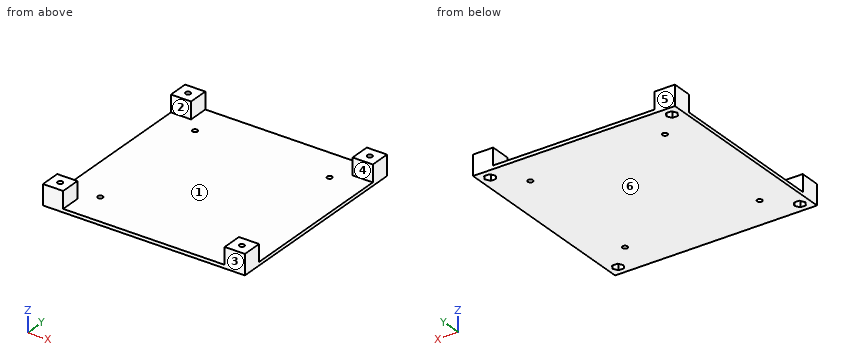
from build123d import *

# Parameters (mm, degrees)
SKETCH_W     = 120
SKETCH_H     = 120
SKETCH_R     = 1.5
PAD_DEPTH    = 2
SKETCH002_W  = 12
SKETCH002_H  = 12
SKETCH002_R  = 1.5
PAD001_DEPTH = 12
POCKET_DEPTH = 9


with BuildPart() as part:
    # Sketch → Pad (new body)
    with BuildSketch(Plane.XY):
        Rectangle(SKETCH_W, SKETCH_H)
        with Locations((-40, 40)):
            Circle(SKETCH_R, mode=Mode.SUBTRACT)
        with Locations((40, 40)):
            Circle(SKETCH_R, mode=Mode.SUBTRACT)
        with Locations((40, -40)):
            Circle(SKETCH_R, mode=Mode.SUBTRACT)
        with Locations((-40, -40)):
            Circle(SKETCH_R, mode=Mode.SUBTRACT)
        with Locations((-54, 54)):
            Circle(SKETCH_R, mode=Mode.SUBTRACT)
        with Locations((54, 54)):
            Circle(SKETCH_R, mode=Mode.SUBTRACT)
        with Locations((54, -54)):
            Circle(SKETCH_R, mode=Mode.SUBTRACT)
        with Locations((-54, -54)):
            Circle(SKETCH_R, mode=Mode.SUBTRACT)
    extrude(amount=PAD_DEPTH)

    # Sketch002 → Pad001 (join)
    with BuildSketch(Plane.XY):
        with Locations((-54, -54)):
            Rectangle(SKETCH002_W, SKETCH002_H)
        with Locations((-54, -54)):
            Circle(SKETCH002_R, mode=Mode.SUBTRACT)
        with Locations((54, -54)):
            Rectangle(SKETCH002_W, SKETCH002_H)
        with Locations((54, -54)):
            Circle(SKETCH002_R, mode=Mode.SUBTRACT)
        with Locations((54, 54)):
            Rectangle(SKETCH002_W, SKETCH002_H)
        with Locations((54, 54)):
            Circle(SKETCH002_R, mode=Mode.SUBTRACT)
        with Locations((-54, 54)):
            Rectangle(SKETCH002_W, SKETCH002_H)
        with Locations((-54, 54)):
            Circle(SKETCH002_R, mode=Mode.SUBTRACT)
    extrude(amount=PAD001_DEPTH)

    # Sketch001 → Pocket (cut)
    with BuildSketch(Plane.XY):
        Polygon((-52.375, 51.185417), (-50.75, 54), (-52.375, 56.814583), (-55.625, 56.814583), (-57.25, 54), (-55.625, 51.185417), align=None)
        Polygon((57.25, 54), (55.625, 56.814583), (52.375, 56.814583), (50.75, 54), (52.375, 51.185417), (55.625, 51.185417), align=None)
        Polygon((-50.75, -54), (-52.375, -51.185417), (-55.625, -51.185417), (-57.25, -54), (-55.625, -56.814583), (-52.375, -56.814583), align=None)
        Polygon((57.25, -54), (55.625, -51.185417), (52.375, -51.185417), (50.75, -54), (52.375, -56.814583), (55.625, -56.814583), align=None)
    extrude(amount=POCKET_DEPTH, mode=Mode.SUBTRACT)


solid = part.part
The model under review builds one solid part; all positions refer to its coordinate system, in mm. Face numbers are marked on the shaded views. A direction names the side the tool comes from. Round coordinates to 2 decimals unless told otherwise and drop trailing zeros. Write each loop counter-clockwise with the first axis right and the second up, starting at its lowest first coordinate (ties: lowest second). Pieces come first, ordered by that corner, then holes. Notation, with made-up numbers: (80, -35.75) -> (106, -35.75) arc R14 ccw to (106, -10.75) -> close; hole circle Ø8 at (-1.5, 44.5). An arc over 180 degrees is marked (long way). Answer as a JSON object with one key per item and string values.
1. To check wall thickness, follow line 1 along Y through (x, z) = (-40, 0.95); line 2 along Y through (x, z) = (54, 11.3). State the ranges of each line that lie inside material, in increasing order.
Results found:
{"line 1": "y = -60 to -41.5, -38.5 to 38.5, 41.5 to 60", "line 2": "y = -60 to -55.5, -52.5 to -48, 48 to 52.5, 55.5 to 60"}
2. The part is to be moulded in two halves that separate along Y. For the marked faces 3, 4, 5 and 6, say which applies: pulls with the +Y half, pulls with the -Y half, needs draft (parallel to the pull), parting line crosses it, or undercut.
Results found:
{"face 3": "pulls with the -Y half", "face 4": "undercut", "face 5": "pulls with the +Y half", "face 6": "needs draft"}
3. We need section C-C on y = -34. State the section outline as (x, z) points, and give its area (3 significant figures).
Results found:
{"outline": "(-60, 0) -> (60, 0) -> (60, 2) -> (-60, 2) -> close", "area": "240 mm^2"}
4. Machinability: for the marked faces 1 and 2, which of the approach directions +Z, -Z, +X, -X, +Y, -Y give a long, thin tool a straight path to every point of the face, cutting with its end or side? Answer none if there is none.
Results found:
{"face 1": "+Z", "face 2": "+Z, +X, -X"}
5. Clearance check with flat-ended pins moving along their axes: pin 1 (3.5 mm diameter, centred on x = -40, y = 40, fed in from +Z); pin 2 (5 mm diameter, centred on x = -54, y = 54, fed in from -Z). State where each tip first meets the part, or that it passes through.
Results found:
{"pin 1": "stops at z = 2", "pin 2": "stops at z = 9"}
6. We need section A-A on x = 54. State the section outline as (y, z) points, and give its area (3 significant figures).
Results found:
{"outline": "(-60, 0) -> (-56.81, 0) -> (-56.81, 9) -> (-55.5, 9) -> (-55.5, 12) -> (-60, 12) -> close; (-52.5, 9) -> (-51.19, 9) -> (-51.19, 0) -> (51.19, 0) -> (51.19, 9) -> (52.5, 9) -> (52.5, 12) -> (48, 12) -> (48, 2) -> (-48, 2) -> (-48, 12) -> (-52.5, 12) -> close; (55.5, 9) -> (56.81, 9) -> (56.81, 0) -> (60, 0) -> (60, 12) -> (55.5, 12) -> close", "area": "361 mm^2"}
7. We need section B-B on z = 6.5. State how many separate pieces and enclosed holes the cut face has, and give its area (3 significant figures).
Results found:
{"separate pieces": "4", "enclosed holes": "4", "area": "466 mm^2"}
